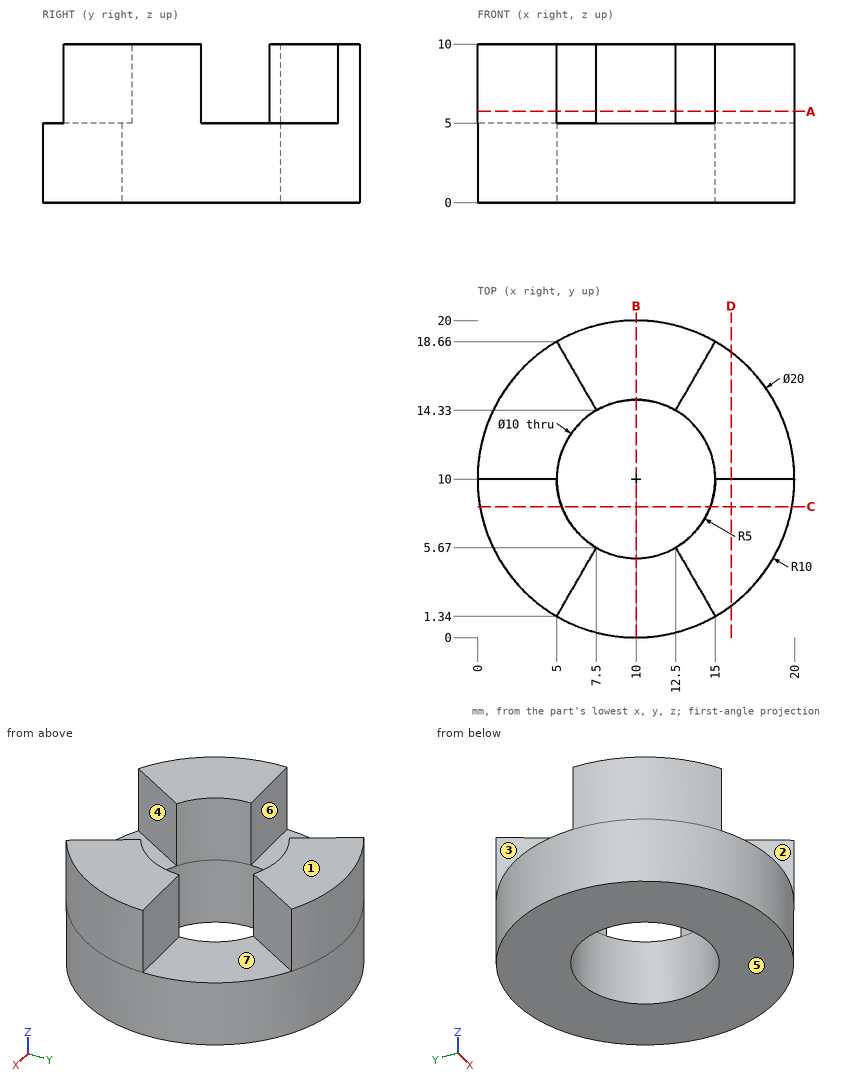
Verification items for this drawing (mm, ordinates from the low corner). A direction names the side the tool comes from. Give positions to 0.01 mm unless a question says otherwise; leave off trailing zeros. Loops run counter-clockwise (first coordinate to the right, second up) from the corner with the lowest first, then second, coordinate; pieces in that order, holes last. Notation, with made-up numbers: M 1.5,68 L 35.5,68 A18 cw 35.5,80 Z; hole C -8.5,-36.5 d4. An arc over 180 degrees is marked long. Answer as a JSON object with one key per item and string values. Group by question number.
Item 1: Sectioned sample at D-D on x = 16. Record the boundary of the cut face in (y, z).
Item 2: Sectioned sample at A-A on z = 5.75. Record the boundary of the cut face in (x, y), plus the area to 3 significant figures.
Item 3: Gauge pin test, flat ends, axial feed: pin 1 (4 mm diameter, centred on x = 13, z = 6, fed in from +Y); pin 2 (1 mm diameter, centred on x = 16, y = 16, fed in from +Z); pin 3 (5.5 mm diameter, centred on x = 1.5, z = 8, fed in from +Y). Record the tip position at first contact, or that the pin passes through.
Item 4: Access from +Z, -Z, +X, -X, +Y, -Y to the whole of each face (thin tool, end or side, straight path). Record for the marked faces 5, 6 and 7.
Item 5: Material ranges on L1, parallel to Y at x = 10, z = 3.45; L2, parallel to Z at x = 8.75, y = 1.75, recorded low to high.
Item 6: Sectioned sample at B-B on x = 10. Record the boundary of the cut face in (y, z), plus the area to 3 significant figures.
Item 7: Sectioned sample at C-C on y = 8.25. Record the boundary of the cut face in (x, z), plus the area to 3 significant figures.
Item 8: Mould release check, pull along X, two halves, no side actions. Record for the marked faces 1, 2, 3 and 4: pulls with the +X half, pulls with the -X half, needs draft (parallel to the pull), parting line crosses it, or undercut.
Findings below:
{
 "1": {"outline": "M 2,0 L 18,0 L 18,5 L 10,5 L 10,10 L 2,10 Z"},
 "2": {"outline": "M 0,10 A10 ccw 5,1.34 L 7.5,5.67 A5 cw 5,10 Z; M 5,18.66 L 7.5,14.33 A5 cw 12.5,14.33 L 15,18.66 A10 ccw Z; M 12.5,5.67 L 15,1.34 A10 ccw 20,10 L 15,10 A5 cw Z", "area": "118 mm2"},
 "3": {"pin 1": "y = 19.95", "pin 2": "z = 5", "pin 3": "y = 10"},
 "4": {"face 5": "-Z, +X, -X, +Y, -Y", "face 6": "+Z, +X, -X, +Y", "face 7": "+Z, +X"},
 "5": {"L1": "0 to 5, 15 to 20", "L2": "0 to 5"},
 "6": {"outline": "M 0,0 L 5,0 L 5,5 L 0,5 Z; M 15,0 L 20,0 L 20,10 L 15,10 Z", "area": "75.0 mm2"},
 "7": {"outline": "M 0.15,0 L 5.32,0 L 5.32,10 L 0.15,10 Z; M 14.68,0 L 19.85,0 L 19.85,10 L 14.68,10 Z", "area": "103 mm2"},
 "8": {"face 1": "needs draft", "face 2": "undercut", "face 3": "pulls with the -X half", "face 4": "undercut"}
}
